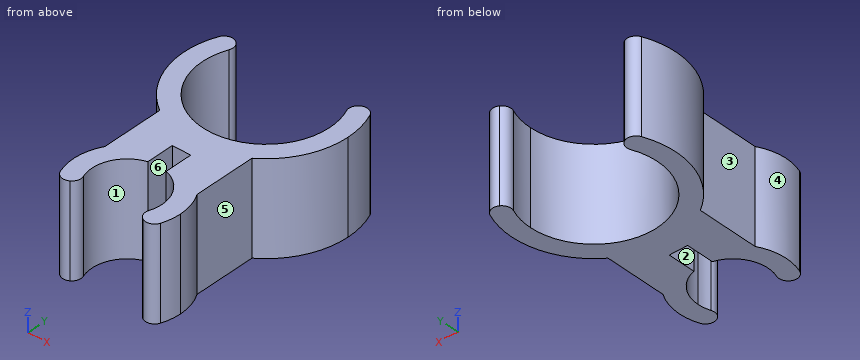
from build123d import *

# Parameters (mm, degrees)
F1_DEPTH = 10
F2_R     = 0.99999


# Not quite as in the source:
# - a fillet or chamfer is up to 0.001 mm smaller than in the source, because OpenCascade refuses the exact size


with BuildPart() as f1:
    # F0 (on Top) → F1 (new body)
    with BuildSketch(Plane.XY):
        with BuildLine():
            ThreePointArc((5.9755752861, 3.45), (6.6648882014, 1.7858514112), (6.9, 0))
            ThreePointArc((6.9, 0), (-1.7858514112, -6.6648882014), (-5.9755752861, 3.45))
            Line((-5.9755752861, 3.45), (-7.7076260937, 4.45))
            ThreePointArc((-7.7076260937, 4.45), (-8.6750314555, -1.9884238095), (-5, -7.3627440537))
            ThreePointArc((-5, -7.3627440537), (0, -8.9), (5, -7.3627440537))
            ThreePointArc((5, -7.3627440537), (7.8647949751, -4.1659332688), (8.9, 0))
            ThreePointArc((8.9, 0), (8.596739854, 2.3034895014), (7.7076260937, 4.45))
            Line((7.7076260937, 4.45), (5.9755752861, 3.45))
        make_face()
        with BuildLine():
            ThreePointArc((5, -7.3627440537), (0, -8.9), (-5, -7.3627440537))
            Line((-5, -7.3627440537), (-5, -14.0606123087))
            ThreePointArc((-5, -14.0606123087), (-3.30506116, -12.233809621), (-1, -11.2868572572))
            Line((-1, -11.2868572572), (-1, -10.333939444))
            Line((-1, -10.333939444), (1, -10.333939444))
            Line((1, -10.333939444), (1, -11.2868572572))
            ThreePointArc((1, -11.2868572572), (3.30506116, -12.233809621), (5, -14.0606123087))
            Line((5, -14.0606123087), (5, -7.3627440537))
        make_face()
        with BuildLine():
            ThreePointArc((-1, -11.2868572572), (-3.30506116, -12.233809621), (-5, -14.0606123087))
            ThreePointArc((-5, -14.0606123087), (-5.7990721969, -17.1037383981), (-4.8916703857, -20.1163377284))
            Line((-4.8916703857, -20.1163377284), (-3.2048874941, -19.0417385117))
            ThreePointArc((-3.2048874941, -19.0417385117), (-3.5447161041, -15.6306980825), (-1, -13.333939444))
            Line((-1, -13.333939444), (-1, -11.2868572572))
        make_face()
        with BuildLine():
            ThreePointArc((5.8, -17), (5.5964274319, -15.4768453788), (5, -14.0606123087))
            ThreePointArc((5, -14.0606123087), (3.30506116, -12.233809621), (1, -11.2868572572))
            Line((1, -11.2868572572), (1, -13.333939444))
            ThreePointArc((1, -13.333939444), (3.0199337741, -14.6934874811), (3.8, -17))
            ThreePointArc((3.8, -17), (3.6481894467, -18.0633502533), (3.2048874941, -19.0417385117))
            Line((3.2048874941, -19.0417385117), (4.8916703857, -20.1163377284))
            ThreePointArc((4.8916703857, -20.1163377284), (5.5682891554, -18.6230082814), (5.8, -17))
        make_face()
    extrude(amount=F1_DEPTH)

    # F2 (radius 1 in the source; OpenCascade refuses exactly that, so slightly less here)
    f2_edges = [f1.edges().sort_by_distance(p)[0] for p in [
        (-7.707626, 4.45, 5),
        (-5.975575, 3.45, 5),
        (5.975575, 3.45, 5),
        (7.707626, 4.45, 5),
        (-4.89167, -20.116338, 5),
        (-3.204887, -19.041739, 5),
        (4.89167, -20.116338, 5),
        (3.204887, -19.041739, 5),
    ]]
    fillet(f2_edges, radius=F2_R)


solid = f1.part
Source: CAD feature listing. Evaluate the final solid. Frame: model axes, mm. Face numbers are marked on the shaded views. A direction names the side the tool comes from. Give positions to 0.01 mm unless a question says otherwise; leave off trailing zeros. Write each loop counter-clockwise with the first axis right and the second up, starting at its lowest first coordinate (ties: lowest second). Pieces come first, ordered by that corner, then holes. Notation, with made-up numbers: M 8,37.25 L 27,37.25 A18 cw 27,61.25 Z; hole C -19.75,-40 d7. An arc over 180 degrees is marked long. Answer as a JSON object with one key per item and string values.
Q1. Ray query, line 1 along X through (y, z) = (0, 7.5); line 2 along Y through (x, z) = (0, 5.75); line 3 along X through (y, z) = (-16.75, 3). Return the intervals inside material, ascending.
Geometry check:
{"line 1": "x = -8.9 to -6.9, 6.9 to 8.9", "line 2": "y = -10.33 to -6.9", "line 3": "x = -5.79 to -3.79, 3.79 to 5.79"}
Q2. Contact query for flat-ended pins moving along their axis: P1, Ø1, axis at y = -5, z = 6, coming from the -X side; P2, Ø5.5, axis at y = -12, z = 3.5, coming from the +X side; P3, Ø5, axis at x = -5.5, y = -9, coming from the +Z side; P4, Ø3.5, axis at y = -11, z = 4.5, coming from the +X side. Output: stop coordinate, or through.
Geometry check:
{"P1": "stops at x = -7.68", "P2": "stops at x = 5.35", "P3": "stops at z = 10", "P4": "stops at x = 5"}
Q3. Cut plane D-D, the plane x = 0. Return the cut outline in (y, z), then the cut area to 3 significant figures.
Geometry check:
{"outline": "M -10.33,0 L -6.9,0 L -6.9,10 L -10.33,10 Z", "area": "34.3 mm^2"}
Q4. Cut plane A-A, the plane y = -13. Return the cut outline in (x, z).
Geometry check:
{"outline": "M -5,0 L -1,0 L -1,10 L -5,10 Z; M 1,0 L 5,0 L 5,10 L 1,10 Z"}
Q5. Cut plane B-B, the plane y = 1.25. Return the cut outline in (x, z).
Geometry check:
{"outline": "M -8.81,0 L -6.79,0 L -6.79,10 L -8.81,10 Z; M 6.79,0 L 8.81,0 L 8.81,10 L 6.79,10 Z"}
Q6. Access query for the marked faces 1, 2 and 3. Directions: +Z, -Z, +X, -X, +Y, -Y. A direction counts if a zero-diameter tool reaches every point of the face in a straight line with its end or side. Return the directions, or none.
Geometry check:
{"face 1": "+Z, -Z", "face 2": "+Z, -Z, -Y", "face 3": "+Z, -Z, -X"}
Q7. Mould query, pull axis X, two halves, no side actions, for the marked faces 4, 5 and 6. Classes: +X half, -X half, draft (parallel to the pull), parting line (faces both ways), or undercut.
Geometry check:
{"face 4": "-X half", "face 5": "+X half", "face 6": "undercut"}
